Check sheet for the modelled part. Datum: model origin and axes. Units: mm. A direction names the side the tool comes from. Give positions to 0.01 mm unless a question says otherwise; leave off trailing zeros. Order: outer loops, then holes, each group sorted by start corner. A loop starts at its lowest first (then second) coordinate and runs counter-clockwise, first axis right, second up.
```python
from build123d import *

# Parameters (mm, degrees)
F0_W     = 7.14375
F0_H     = 4.7625
F0_R     = 0.635
F0_W_2   = 68.4589182
F1_DEPTH = 2.1166666667
F2_DEPTH = 4.2333333333
F3_START = 4.2333333333
F3_DEPTH = 2.1166666667


with BuildPart() as f1:
    # F0 (on Top) → F1 (new body)
    with BuildSketch(Plane.XY):
        with Locations((-37.8013341, 0)):
            Rectangle(F0_W, F0_H)
        with Locations((-37.8013341, 0)):
            Circle(F0_R, mode=Mode.SUBTRACT)
        Rectangle(F0_W_2, F0_H)
        with Locations((37.8013341, 0)):
            Rectangle(F0_W, F0_H)
        with Locations((37.8013341, 0)):
            Circle(F0_R, mode=Mode.SUBTRACT)
    extrude(amount=F1_DEPTH)

    # F0 (on Top) → F2 (join)
    with BuildSketch(Plane.XY):
        Rectangle(F0_W_2, F0_H)
    extrude(amount=F2_DEPTH)

    # F0 (on Top) → F3 (join)
    with BuildSketch(Plane.XY.offset(F3_START)):
        with Locations((-37.8013341, 0)):
            Rectangle(F0_W, F0_H)
        with Locations((-37.8013341, 0)):
            Circle(F0_R, mode=Mode.SUBTRACT)
        Rectangle(F0_W_2, F0_H)
    extrude(amount=F3_DEPTH)


solid = f1.part
```
Q1. Go/stop test with a flat-tipped pin: P1, Ø1.1, axis at y = 0.5, z = 3, coming from the -X side. Record where the tip stops, or that it passes through.
Q2. Sectioned sample at A-A, the plane z = 5.5. Record the cut outline in (x, y) (3 decimals), plus the area to 3 significant figures.
Q3. Tool access check on faces 4 (the flat face through (-34.229, 0, 3)), 5 (the flat face through (-41.373, 0, 5)), 6 (the flat face through (37, 0, 2.117)). Record the directions out of +Z, -Z, +X, -X, +Y, -Y that give a thin tool (end or side, any length) a straight path to the whole face; none if there is none.
Q4. Draft check along X on faces 1 (the flat face through (34.229, 0, 4)), 2 (the flat face through (-39, 0, 2.117)), 3 (the cylindrical face through (-38.27, 0.43, 1.04)). Enter one of: pulls with the +X half, pulls with the -X half, needs draft (parallel to the pull), parting line crosses it, or undercut.
Q5. Material ranges on line 1 (X direction, y = 0.05, z = 5.25); line 2 (X direction, y = -1.7, z = 5.25); line 3 (Z direction, x = 38.5, y = -0.35), recorded low to high.
Filled in:
1. P1: stops at x = -34.23
2. outline: (-41.373, -2.381) - (34.229, -2.381) - (34.229, 2.381) - (-41.373, 2.381) - close; hole circle Ø1.27 at (-37.801, 0)
2. area: 359 mm2
3. face 4: -X, +Y, -Y
3. face 5: +Z, -Z, -X, +Y, -Y
3. face 6: +Z, +X, +Y, -Y
4. face 1: pulls with the +X half
4. face 2: needs draft
4. face 3: undercut
5. line 1: x = -41.37 to -38.43, -37.17 to 34.23
5. line 2: x = -41.37 to 34.23
5. line 3: z = 0 to 2.12
